from build123d import *

# Parameters (mm, degrees)
CROQUIS1_W              = 42
CROQUIS1_H              = 42
SALIENTE_EXTRUIR1_DEPTH = 6
CROQUIS2_R              = 1.5
CROQUIS2_R_2            = 12
CORTAR_EXTRUIR2_DEPTH   = 6
CROQUIS4_R              = 2.05
CORTAR_EXTRUIR3_DEPTH   = 3
CROQUIS5_R              = 2.05
CORTAR_EXTRUIR4_DEPTH   = 3
SALIENTE_EXTRUIR2_START = 5
CROQUIS6_R              = 2.95
CROQUIS6_R_2            = 2.05
SALIENTE_EXTRUIR2_DEPTH = 5
SALIENTE_EXTRUIR3_START = 5
CROQUIS7_R              = 2.95
CROQUIS7_R_2            = 2.05
SALIENTE_EXTRUIR3_DEPTH = 5


with BuildPart() as part:
    # Croquis1 → Saliente-Extruir1 (new body)
    with BuildSketch(Plane(origin=(0, 0, 0), x_dir=(1, 0, 0), z_dir=(0, 1, 0))):
        Rectangle(CROQUIS1_W, CROQUIS1_H)
    extrude(amount=SALIENTE_EXTRUIR1_DEPTH)

    # Croquis2 → Cortar-Extruir2 (cut)
    with BuildSketch(Plane(origin=(0, 6, 0), x_dir=(1, 0, 0), z_dir=(0, 1, 0))):
        with Locations(Location((-15.5, -14.5, 0), (0, 0, 270))):
            Circle(CROQUIS2_R)
        with Locations(Location((14.5, -14.5, 0), (0, 0, 270))):
            Circle(CROQUIS2_R)
        with Locations(Location((14.5, 14.5, 0), (0, 0, 270))):
            Circle(CROQUIS2_R)
        with Locations(Location((-15.5, 14.5, 0), (0, 0, 270))):
            Circle(CROQUIS2_R)
        with Locations(Location((0, 0, 0), (0, 0, 270))):
            Circle(CROQUIS2_R_2)
    extrude(amount=-CORTAR_EXTRUIR2_DEPTH, mode=Mode.SUBTRACT)

    # Croquis4 → Cortar-Extruir3 (cut)
    with BuildSketch(Plane(origin=(21, 0, 0), x_dir=(0, 0, -1), z_dir=(1, 0, 0))):
        with Locations((12, 3)):
            Circle(CROQUIS4_R)
        with Locations((0, 3)):
            Circle(CROQUIS4_R)
    extrude(amount=-CORTAR_EXTRUIR3_DEPTH, mode=Mode.SUBTRACT)

    # Croquis5 → Cortar-Extruir4 (cut)
    with BuildSketch(Plane.ZY.offset(21)):
        with Locations((-12, 3.206908841)):
            Circle(CROQUIS5_R)
        with Locations((0, 3.206908841)):
            Circle(CROQUIS5_R)
    extrude(amount=-CORTAR_EXTRUIR4_DEPTH, mode=Mode.SUBTRACT)

    # Croquis6 → Saliente-Extruir2 (add)
    with BuildSketch(Plane(origin=(21, 0, 0), x_dir=(0, 0, -1), z_dir=(1, 0, 0)).offset(SALIENTE_EXTRUIR2_START)):
        with Locations(Location((0, 3, 0), (0, 0, 180))):
            Circle(CROQUIS6_R)
        with Locations((0, 3)):
            Circle(CROQUIS6_R_2, mode=Mode.SUBTRACT)
    extrude(amount=-SALIENTE_EXTRUIR2_DEPTH)

    # Croquis7 → Saliente-Extruir3 (add)
    with BuildSketch(Plane.ZY.offset(21).offset(SALIENTE_EXTRUIR3_START)):
        with Locations(Location((0, 3.206908841, 0), (0, 0, 108.771300902))):
            Circle(CROQUIS7_R)
        with Locations((0, 3.206908841)):
            Circle(CROQUIS7_R_2, mode=Mode.SUBTRACT)
    extrude(amount=-SALIENTE_EXTRUIR3_DEPTH)


solid = part.part
Verification items for the finished model (mm, model axes). A direction names the side the tool comes from. Give positions to 0.01 mm unless a question says otherwise; leave off trailing zeros. Order: outer loops, then holes, each group sorted by start corner. A loop starts at its lowest first (then second) coordinate and runs counter-clockwise, first axis right, second up. Notation, with made-up numbers: (56, 85) -> (110, 85) arc R24 cw to (110, 98) -> close; hole circle Ø10 at (-16, 34.5). An arc over 180 degrees is marked (long way). Answer as CSV lines item,"result".
Q1. Sectioned sample at B-B on x = 14.5. Record the cut outline in (y, z).
Solutions:
outline,"(0, -21) -> (6, -21) -> (6, -16) -> (0, -16) -> close; (0, -13) -> (6, -13) -> (6, 13) -> (0, 13) -> close; (0, 16) -> (6, 16) -> (6, 21) -> (0, 21) -> close"
Q2. Sectioned sample at A-A on z = 0. Record the cut outline in (x, y).
Solutions:
outline,"(-26, 0.26) -> (-21, 0.26) -> (-21, 0) -> (-12, 0) -> (-12, 6) -> (-21, 6) -> (-21, 6.16) -> (-26, 6.16) -> (-26, 5.26) -> (-18, 5.26) -> (-18, 1.16) -> (-26, 1.16) -> close; (12, 0) -> (21, 0) -> (21, 0.05) -> (26, 0.05) -> (26, 0.95) -> (18, 0.95) -> (18, 5.05) -> (26, 5.05) -> (26, 5.95) -> (21, 5.95) -> (21, 6) -> (12, 6) -> close"
Q3. Access from +Z, -Z, +X, -X, +Y, -Y to the whole of each face (thin tool, end or side, straight path). Record for faces 5 (the flat face through (18, 3, -12)), 6 (the flat face through (0, 3, 21)), 7 (the flat face through (-18, 3, -12)).
Solutions:
face 5,"+X"
face 6,"+Z, +X, -X, +Y, -Y"
face 7,"-X"
Q4. Scan lines: probe 1 along X at (y, z) = (2.6, 14.5); probe 2 along Y at (x, z) = (19.35, -12); probe 3 along Y at (x, z) = (21.5, 0). Record each from-to range of solid material in increasing order.
Solutions:
probe 1,"x = -21 to -17, -14 to 13, 16 to 21"
probe 2,"y = 0 to 0.95, 5.05 to 6"
probe 3,"y = 0.05 to 0.95, 5.05 to 5.95"
Q5. Release check for a two-part mould opening along Z. For faces 1 (the cylindrical face through (3.604, 3.042, 11.446)), 2 (the flat face through (0, 3, -21)), 3 (the flat face through (26, 1, 1)), 4 (the cylindrical face through (-23.54, 5.59, -1.74)) record: +Z half, -Z half, draft (parallel to the pull), parting line (faces both ways), or undercut.
Solutions:
face 1,"undercut"
face 2,"-Z half"
face 3,"draft"
face 4,"parting line"
Q6. Depth check by flat-ended pin: pin 1 (2 mm diameter, centred on y = 4, z = -1, fed in from -X); pin 2 (2.5 mm diameter, centred on y = 3, z = -12, fed in from +X); pin 3 (4 mm diameter, centred on x = 14.5, z = 14.5, fed in from +Y); pin 4 (2 mm diameter, centred on y = 3.5, z = -13, fed in from +X). Enter the tip coordinate at first touch or a pass-through.
Solutions:
pin 1,"stops at x = -26"
pin 2,"stops at x = 18"
pin 3,"stops at y = 6"
pin 4,"stops at x = 21"
Q7. Sectioned sample at D-D on x = 0. Record the cut outline in (y, z).
Solutions:
outline,"(0, -21) -> (6, -21) -> (6, -12) -> (0, -12) -> close; (0, 12) -> (6, 12) -> (6, 21) -> (0, 21) -> close"
Q8. Sectioned sample at C-C on z = 14.5. Record the cut outline in (x, y).
Solutions:
outline,"(-21, 0) -> (-17, 0) -> (-17, 6) -> (-21, 6) -> close; (-14, 0) -> (13, 0) -> (13, 6) -> (-14, 6) -> close; (16, 0) -> (21, 0) -> (21, 6) -> (16, 6) -> close"
